Geometry: final body of the model. Coordinates: model frame, mm. Face numbers are marked on the shaded views. A direction names the side the tool comes from. Coordinates: 2 decimals unless noted, no trailing zeros. Loops run counter-clockwise (first coordinate to the right, second up) from the corner with the lowest first, then second, coordinate; pieces in that order, holes last. Notation, with made-up numbers: M -22,62 L 0,62 A15 cw 0,79 Z; hole C 70,40.25 d1. An arc over 180 degrees is marked long. Write item = value, one per line. Start each with the question number.
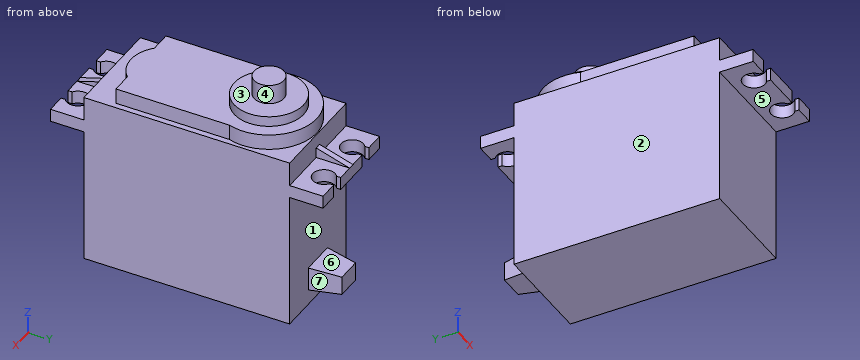
Autodesk Inventor part; units mm, degrees
ref_plane "YZ Plane" through (0, 0, 0) normal (1, 0, 0) x (0, 1, 0)
ref_plane "XZ Plane" through (0, 0, 0) normal (0, 1, 0) x (-1, 0, 0)
ref_plane "XY Plane" through (0, 0, 0) normal (0, 0, 1) x (1, 0, 0)
sketch "Sketch1" plane through (0, 0, 0) normal (0, 0, 1) x (1, 0, 0)
  line L0 (-14, 0) -> (14, 0)
  line L1 (0, 28) -> (0, -28)
  line L2 (-10, 20) -> (10, 20)
  line L3 (10, 20) -> (10, -20)
  line L4 (10, -20) -> (-10, -20)
  line L5 (-10, -20) -> (-10, 20)
  point P0 (0, 0)
  dimension "d0" = 20
  dimension "d1" = 40
extrude "Extrusion1" add sketch "Sketch1" along normal blind 7.2 and the other way blind 26.5
sketch "Sketch2" plane through (0, 0, 0) normal (0, 0, 1) x (1, 0, 0)
  line L0 (-14, 0) -> (14, 0)
  line L1 (0, 28) -> (0, -28)
  line L2 (-10, 20) -> (-10, -20)
  line L3 (10, -20) -> (10, 20)
  line L4 (-10, 26.5) -> (10, 26.5)
  line L5 (10, 26.5) -> (10, -26.5)
  line L6 (10, -26.5) -> (-10, -26.5)
  line L7 (-10, -26.5) -> (-10, 26.5)
  point P0 (0, 0)
  dimension "d6" = 53
extrude "Extrusion2" add sketch "Sketch2" along normal blind 2.5
sketch "Sketch3" plane through (0, 0, 0) normal (0, 0, 1) x (1, 0, 0)
  line L0 (0, 37.1) -> (0, -37.1)
  line L1 (-14, 0) -> (14, 0)
  line L2 (-5, 23.925) -> (5, 23.925) construction
  line L3 (5, 23.925) -> (5, -23.925) construction
  line L4 (5, -23.925) -> (-5, -23.925) construction
  line L5 (-5, -23.925) -> (-5, 23.925) construction
  point P0 (0, 0)
  dimension "d9" = 47.85
  dimension "d10" = 10
hole "Hole1" at (5, 23.925, 0) at (-5, 23.925, 0) at (-5, -23.925, 0) at (5, -23.925, 0) direction (0, 0, 1) diameter 4.35 depth 8 tip angle 118
sketch "Sketch4" plane through (0, 0, 0) normal (0, 0, 1) x (1, 0, 0)
  line L0 (-14, 0) -> (14, 0)
  line L1 (0, 37.1) -> (0, -37.1)
  line L2 (10, 26.5) -> (-10, 26.5)
  line L3 (-10, -26.5) -> (10, -26.5)
  circle A0 centre (-5, 23.925) radius 2.175
  circle A1 centre (5, 23.925) radius 2.175
  circle A2 centre (-5, -23.925) radius 2.175
  circle A3 centre (5, -23.925) radius 2.175
  line L4 (-6.25, -23.925) -> (-3.75, -23.925)
  line L5 (-3.75, -23.925) -> (-3.75, -26.5)
  line L6 (-3.75, -26.5) -> (-6.25, -26.5)
  line L7 (-6.25, -26.5) -> (-6.25, -23.925)
  line L8 (6.25, -23.925) -> (3.75, -23.925)
  line L9 (3.75, -23.925) -> (3.75, -26.5)
  line L10 (3.75, -26.5) -> (6.25, -26.5)
  line L11 (6.25, -26.5) -> (6.25, -23.925)
  line L12 (-10, 26.5) -> (10, 26.5)
  line L13 (6.25, 26.5) -> (3.75, 26.5)
  line L14 (3.75, 26.5) -> (3.75, 23.925)
  line L15 (3.75, 23.925) -> (6.25, 23.925)
  line L16 (6.25, 23.925) -> (6.25, 26.5)
  line L17 (-3.75, 26.5) -> (-6.25, 26.5)
  line L18 (-6.25, 26.5) -> (-6.25, 23.925)
  line L19 (-6.25, 23.925) -> (-3.75, 23.925)
  line L20 (-3.75, 23.925) -> (-3.75, 26.5)
  point P0 (0, 0)
  dimension "d18" = 2.5
  dimension "d19" = 2.5
  dimension "d20" = 2.5
  dimension "d21" = 2.5
extrude "Extrusion3" cut sketch "Sketch4" along normal through all contours L9 A3 L11 L3 | L3 L7 A2 L5 | L2 L16 A1 L14 | L20 A0 L18 L2 | A1 L16 L15 L14 | L20 L19 L18 A0 | A2 L7 L4 L5 | L9 L8 L11 A3 picked at (4.9114, 24.6446) picked at (-5.0886, 24.6446) picked at (-5.0886, -24.6446) picked at (4.9114, -24.6446)
sketch "Sketch5" plane through (0, 0, 0) normal (1, 0, 0) x (0, 1, 0)
  line L0 (20, 2.5) -> (26.5, 2.5)
  line L1 (20, 7.2) -> (20, 2.5)
  line L2 (26.5, 2.5) -> (20, 2.5)
  line L3 (20, 2.5) -> (20, 4.5)
  line L4 (20, 4.5) -> (26.5, 2.5)
  point P0 (0, 0)
  dimension "d24" = 2
extrude "Extrusion4" add sketch "Sketch5" along normal mid plane 1.2
mirror "Mirror1" about plane through (0, 0, 0) normal (0, 1, 0) of "Extrusion4"
sketch "Sketch6" plane through (0, 0, 7.2) normal (0, 0, 1) x (1, 0, 0)
  line L0 (0, 37.1) -> (0, -37.1)
  line L1 (-14, 0) -> (14, 0)
  circle A0 centre (0, 10.5) radius 6.75
  line L2 (-10, -20) -> (10, -20)
  point P0 (0, 0)
  dimension "d27" = 30.5
  dimension "d28" = 13.5
extrude "Extrusion5" add sketch "Sketch6" along normal blind 5
sketch "Sketch7" plane through (0, 0, 7.2) normal (0, 0, 1) x (1, 0, 0)
  circle A0 centre (0, 10.5) radius 6.75
  circle A1 centre (0, 10.5) radius 9.3
  point P0 (0, 0)
  dimension "d31" = 18.6
extrude "Extrusion6" add sketch "Sketch7" along normal blind 3
sketch "Sketch8" plane through (0, 0, 7.2) normal (0, 0, 1) x (1, 0, 0)
  line L0 (-14, 0) -> (14, 0)
  line L1 (0, 37.1) -> (0, -37.1)
  circle A0 centre (0, 10.5) radius 9.3
  line L2 (-8.85, 10.5) -> (8.85, 10.5)
  line L3 (8.85, 10.5) -> (8.85, -14.4)
  line L4 (8.85, -14.4) -> (-8.85, -14.4)
  line L5 (-8.85, -14.4) -> (-8.85, 10.5)
  line L6 (10, 20) -> (-10, 20)
  point P0 (0, 0)
  dimension "d34" = 17.7
  dimension "d35" = 34.4
extrude "Extrusion7" add sketch "Sketch8" along normal blind 3 contours L5 A0 L1 L0 | L0 L1 L4 L5 | L1 A0 L3 L0 | L0 L3 L4 L1 | L5 L2 L1 A0 | L1 L2 L3 A0 picked at (-5.9, 9.5474) picked at (5.9, 9.5474)
sketch "Sketch9" plane through (0, 0, 7.2) normal (0, 0, 1) x (1, 0, 0)
  line L0 (0, 37.1) -> (0, -37.1)
  line L1 (10, 20) -> (-10, 20)
  line L2 (-8.85, -14.4) -> (8.85, -14.4)
  arc A0 (-4.8, -14.4) -> (4.8, -14.4) centre (0, -9.4673) ccw
  point P0 (0, 0)
  dimension "d38" = 9.6
  dimension "d39" = 36.35
extrude "Extrusion8" add sketch "Sketch9" along normal blind 3
sketch "Sketch10" plane through (-10, 20, -26.5) normal (0, 1, 0) x (1, 0, 0)
  line L0 (0, 0) -> (20, 0)
  line L1 (10, 7.74) -> (10, -46.44)
  line L2 (0, -26.5) -> (20, -26.5)
  line L3 (20, -26.5) -> (20, 0)
  line L4 (0, 0) -> (20, 0)
  line L5 (0, 0) -> (0, -26.5)
  line L6 (6.6, -7.6) -> (13.4, -7.6)
  line L7 (13.4, -7.6) -> (13.4, -3)
  line L8 (13.4, -3) -> (6.6, -3)
  line L9 (6.6, -3) -> (6.6, -7.6)
  point P0 (10, -26.5)
  dimension "d42" = 3
  dimension "d43" = 4.6
  dimension "d44" = 6.8
extrude "Extrusion9" add sketch "Sketch10" along normal blind 6 contours L8 L7 L6 L1 | L1 L6 L9 L8
chamfer "Chamfer1" distance 6 distance2 1 1 edges at (3.4, 26, -21.2) measured on face at (3.4, 22, -20.4333)
chamfer "Chamfer2" distance 6 distance2 1 1 edges at (-3.4, 26, -21.2) measured on face at (-3.4, 22, -21.9667)
chamfer "Chamfer3" distance 6 distance2 0.5 1 edges at (0, 26, -18.9) measured on face at (0.8002, 22.0003, -18.9)
chamfer "Chamfer4" distance 6 distance2 0.5 1 edges at (0, 26, -23.5) measured on face at (0.8002, 22.0003, -23.5)
sketch "Sketch11" plane through (0, 10.5, 12.2) normal (0, 0, 1) x (1, 0, 0)
  circle A0 centre (0, 0) radius 6.75
  circle A1 centre (0, 0) radius 2.9
  point P0 (0, -10.5)
  dimension "d59" = 5.8
extrude "Extrusion10" add sketch "Sketch11" along normal blind 3.8 contours A1
equation "\"d19\" = d18"
equation "\"d20\" = d18"
equation "\"d21\" = d18"
properties part number "servo motor HS-7955TG"
Item 1: Line query: line 1 (Y direction, x = 5, z = 1.45); line 2 (Y direction, x = 9.25, z = -13); line 3 (X direction, y = -6, z = 9). Output: solid intervals per line, ascending. Write a range as from..to.
Item 2: First-contact query: pin 1 (4 mm diameter, centred on x = 0.5, z = -22, fed in from +Y); pin 2 (1.5 mm diameter, centred on x = 7.5, z = 8.5, fed in from -Y); pin 3 (2 mm diameter, centred on x = 4, y = 24, fed in from +Z) (1 decimal); pin 4 (0.6 mm diameter, centred on y = -22, z = 3.5, fed in from +X). Flat tips, straight axial feed; report the tip coordinate or a pass-through.
Item 3: Reachability of the marked faces 4, 5, 6 and 7 from +Z, -Z, +X, -X, +Y, -Y: full face, straight path, thin tool, end or side. Return the list, or none.
Item 4: Section query D-D (z = -18). Return the cut outline in (x, y).
Item 5: Section query C-C (y = 10.5). Return the cut outline in (x, z).
Item 6: Pull-direction query (Z, two-part tool) for the marked faces 1, 2 and 3; classes: released by +Z, released by -Z, zero draft, split by the parting line, or undercut.
Item 7: Section query A-A (y = -23). Return the cut outline in (x, z).
Verdict:
q1.line_1 = -21.75..21.75
q1.line_2 = -20..20
q1.line_3 = -8.85..8.85
q2.pin_1 = 26
q2.pin_2 = -14.4
q2.pin_3 = through
q2.pin_4 = 0.6
q3.face_4 = +Z
q3.face_5 = -Z, +X, -X, -Y
q3.face_6 = +X, -X, +Y
q3.face_7 = -Z, +X, +Y
q4.outline = M -10,-20 L 10,-20 L 10,20 L -10,20 Z
q5.outline = M -10,-26.5 L 10,-26.5 L 10,7.2 L 9.3,7.2 L 9.3,10.2 L 6.75,10.2 L 6.75,12.2 L 2.9,12.2 L 2.9,16 L -2.9,16 L -2.9,12.2 L -6.75,12.2 L -6.75,10.2 L -9.3,10.2 L -9.3,7.2 L -10,7.2 Z
q6.face_1 = undercut
q6.face_2 = zero draft
q6.face_3 = released by +Z
q7.outline = M -10,0 L -6.97,0 L -6.97,2.5 L -10,2.5 Z; M -3.03,0 L 3.03,0 L 3.03,2.5 L 0.6,2.5 L 0.6,3.58 L -0.6,3.58 L -0.6,2.5 L -3.03,2.5 Z; M 6.97,0 L 10,0 L 10,2.5 L 6.97,2.5 Z
